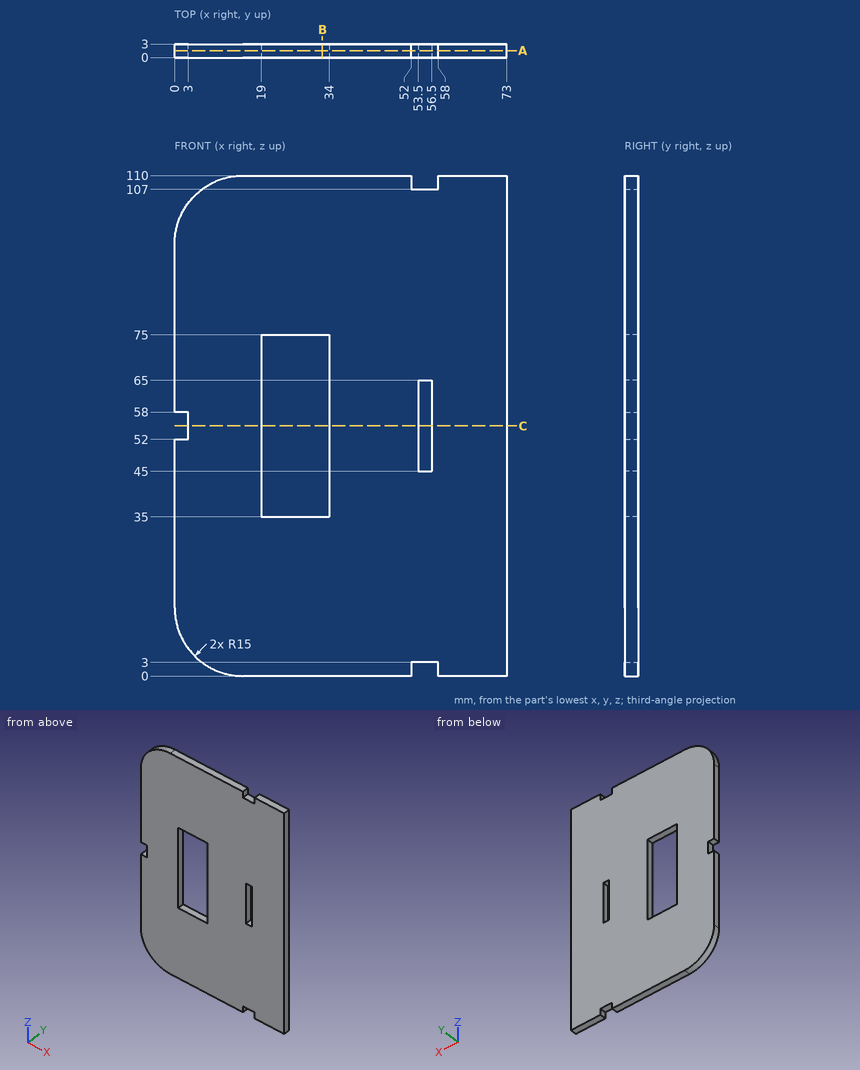
Study the drawing (mm; zero at the part's minimum x, y, z) and answer. Give positions to 0.01 mm unless a question says otherwise; leave off trailing zeros. Order: outer loops, then holes, each group sorted by start corner. A loop starts at its lowest first (then second) coordinate and runs counter-clockwise, first axis right, second up.
1. Straight lines are drawn through the part: L1, parallel to X at y = 1.85, z = 62.5; L2, parallel to X at y = 0.45, z = 53.5; L3, parallel to Z at x = 55, y = 2.6. For each, find the intervals that lie inside material, in ascending order.
Result sheet:
L1: x = 0 to 19, 34 to 53.5, 56.5 to 73
L2: x = 3 to 19, 34 to 53.5, 56.5 to 73
L3: z = 3 to 45, 65 to 107
2. Section B-B, the plane x = 32.5 is taken. Determine the outline of the cut face in (y, z), and give its area (3 significant figures).
Result sheet:
outline: (0, 0) - (3, 0) - (3, 35) - (0, 35) - close; (0, 75) - (3, 75) - (3, 110) - (0, 110) - close
area: 210 mm2
3. Section A-A, the plane y = 1.55 is taken. Determine the outline of the cut face in (x, z), and give its area (3 significant figures).
Result sheet:
outline: (0, 15) arc R15 ccw to (15, 0) - (52, 0) - (52, 3) - (58, 3) - (58, 0) - (73, 0) - (73, 110) - (58, 110) - (58, 107) - (52, 107) - (52, 110) - (15, 110) arc R15 ccw to (0, 95) - (0, 58) - (3, 58) - (3, 52) - (0, 52) - close; hole (19, 35) - (34, 35) - (34, 75) - (19, 75) - close; hole (53.5, 45) - (56.5, 45) - (56.5, 65) - (53.5, 65) - close
area: 7,220 mm2
4. Section C-C, the plane z = 55 is taken. Determine the outline of the cut face in (x, y), and give its area (3 significant figures).
Result sheet:
outline: (3, 0) - (19, 0) - (19, 3) - (3, 3) - close; (34, 0) - (53.5, 0) - (53.5, 3) - (34, 3) - close; (56.5, 0) - (73, 0) - (73, 3) - (56.5, 3) - close
area: 156 mm2
5. Each of these flat-tipped pins is pushed along its axis until it touches: P1, Ø4, axis at x = 34, z = 80, coming from the -Y side; P2, Ø1.5, axis at x = 56, y = 2, coming from the +Z side; P3, Ø0.9, axis at y = 2, z = 108, coming from the -X side; P4, Ø0.9, axis at y = 1.5, z = 56.5, coming from the -X side. Where does it stop, or does it pass through?
Result sheet:
P1: stops at y = 0
P2: stops at z = 107
P3: stops at x = 6.78
P4: stops at x = 3
